Read the model definition and answer for the solid it produces. Units are mm, in the model's axes. Face numbers are marked on the shaded views. Give positions to 0.01 mm unless a question says otherwise; leave off trailing zeros. Order: outer loops, then holes, each group sorted by start corner. A loop starts at its lowest first (then second) coordinate and runs counter-clockwise, first axis right, second up. Notation, with made-up numbers: (54, -5) -> (100, -5) arc R10 ccw to (100, 10) -> close; hole circle Ø6 at (29.5, -35). An arc over 180 degrees is marked (long way). Use one line per item in the form item = value.
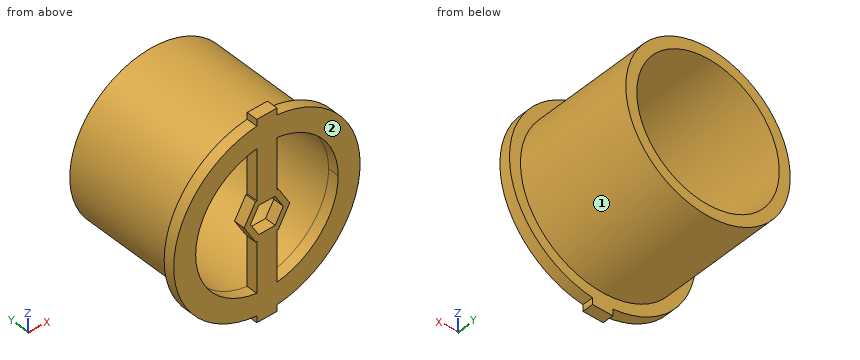
```python
from build123d import *

# Parameters (mm, degrees)
BOSS_EXTRUDE3_DEPTH = 5
CUT_EXTRUDE1_DEPTH  = 6
SKETCH1_R           = 37.5
SKETCH1_R_2         = 32.5
BOSS_EXTRUDE4_DEPTH = 60


with BuildPart() as part:
    # Sketch4 → Boss-Extrude3 (new body)
    with BuildSketch(Plane(origin=(0, 0, 0), x_dir=(1, 0, 0), z_dir=(0, 1, 0))):
        with BuildLine():
            Line((-4.63627719, -42.246360007), (-4.63627719, -45.246360007))
            Line((-4.63627719, -45.246360007), (4.63627719, -45.246360007))
            Line((4.63627719, -45.246360007), (4.63627719, -42.246360007))
            ThreePointArc((4.63627719, -42.246360007), (42.5, 0), (4.63627719, 42.246360007))
            Line((4.63627719, 42.246360007), (4.63627719, 45.246360007))
            Line((4.63627719, 45.246360007), (-4.63627719, 45.246360007))
            Line((-4.63627719, 45.246360007), (-4.63627719, 42.246360007))
            ThreePointArc((-4.63627719, 42.246360007), (-42.5, 0), (-4.63627719, -42.246360007))
        make_face()
        with BuildLine():
            Line((-4.63627719, 32.167606902), (-4.63627719, 9))
            Line((-4.63627719, 9), (-5.196152423, 9))
            Line((-5.196152423, 9), (-10.392304845, 0))
            Line((-10.392304845, 0), (-5.196152423, -9))
            Line((-5.196152423, -9), (-4.63627719, -9))
            Line((-4.63627719, -9), (-4.63627719, -32.167606902))
            ThreePointArc((-4.63627719, -32.167606902), (-32.5, 0), (-4.63627719, 32.167606902))
        make_face(mode=Mode.SUBTRACT)
        with BuildLine():
            Line((4.63627719, 32.167606902), (4.63627719, 9))
            Line((4.63627719, 9), (5.196152423, 9))
            Line((5.196152423, 9), (10.392304845, 0))
            Line((10.392304845, 0), (5.196152423, -9))
            Line((5.196152423, -9), (4.63627719, -9))
            Line((4.63627719, -9), (4.63627719, -32.167606902))
            ThreePointArc((4.63627719, -32.167606902), (32.5, 0), (4.63627719, 32.167606902))
        make_face(mode=Mode.SUBTRACT)
    extrude(amount=BOSS_EXTRUDE3_DEPTH)

    # Sketch7 → Cut-Extrude1 (cut, through all)
    with BuildSketch(Plane(origin=(0, 0, 0), x_dir=(-1, 0, 0), z_dir=(0, -1, 0))):
        Polygon((-7.505553499, 0), (-3.75277675, -6.5), (3.75277675, -6.5), (7.505553499, 0), (3.75277675, 6.5), (-3.75277675, 6.5), align=None)
    extrude(amount=-CUT_EXTRUDE1_DEPTH, mode=Mode.SUBTRACT)

    # Sketch1 → Boss-Extrude4 (add)
    with BuildSketch(Plane(origin=(0, 0, 0), x_dir=(1, 0, 0), z_dir=(0, 1, 0))):
        Circle(SKETCH1_R)
        Circle(SKETCH1_R_2, mode=Mode.SUBTRACT)
    extrude(amount=BOSS_EXTRUDE4_DEPTH)


solid = part.part
```
Item 1: Determine the mould class of the marked faces 1 and 2 for opening direction X: +X half, -X half, draft (parallel to the pull), parting line (faces both ways), or undercut.
Checks:
face_1 = parting line
face_2 = draft
Item 2: The part is cut by section C-C on y = 18. Give the vertices of the cut face in (x, z).
Checks:
outline = circle Ø75 at (0, 0); hole circle Ø65 at (0, 0)
Item 3: The part is cut by section B-B on z = -23. Give the vertices of the cut face in (x, y), and give its area (3 significant figures).
Checks:
outline = (-35.74, 0) -> (-22.96, 0) -> (-22.96, 60) -> (-29.62, 60) -> (-29.62, 5) -> (-35.74, 5) -> close; (-4.64, 0) -> (4.64, 0) -> (4.64, 5) -> (-4.64, 5) -> close; (22.96, 0) -> (35.74, 0) -> (35.74, 5) -> (29.62, 5) -> (29.62, 60) -> (22.96, 60) -> close
area = 906 mm²
Item 4: The part is cut by section D-D on x = 16.5. Give the vertices of the cut face in (y, z), and give its area (3 significant figures).
Checks:
outline = (0, -39.17) -> (5, -39.17) -> (5, -33.67) -> (60, -33.67) -> (60, -28) -> (0, -28) -> close; (0, 28) -> (60, 28) -> (60, 33.67) -> (5, 33.67) -> (5, 39.17) -> (0, 39.17) -> close
area = 736 mm²
Item 5: The part is cut by section A-A on x = 0. Give the vertices of the cut face in (y, z).
Checks:
outline = (0, -45.25) -> (5, -45.25) -> (5, -37.5) -> (60, -37.5) -> (60, -32.5) -> (5, -32.5) -> (5, -6.5) -> (0, -6.5) -> close; (0, 6.5) -> (5, 6.5) -> (5, 32.5) -> (60, 32.5) -> (60, 37.5) -> (5, 37.5) -> (5, 45.25) -> (0, 45.25) -> close
Item 6: Straight lines are drawn through the part: L1, parallel to Z at x = 0, y = 44; L2, parallel to Z at x = 9, y = 57. For each, find the intervals that lie inside material, in ascending order. Write a range as from..to.
Checks:
L1 = -37.5..-32.5, 32.5..37.5
L2 = -36.4..-31.23, 31.23..36.4
Item 7: Given pin 1 Ø12 at (y, z) = (37, 36) entering from -X; pin 2 Ø6 at (x, y) = (-20, 37) entering from +Z; pin 3 Ø12 at (x, y) = (-28.5, 46.5) entering from -Z, each flat-ended and moving along its own axis, determine where each tip first touches the part or whether it passes through.
Checks:
pin_1 = -22.5
pin_2 = 33.43
pin_3 = -30
